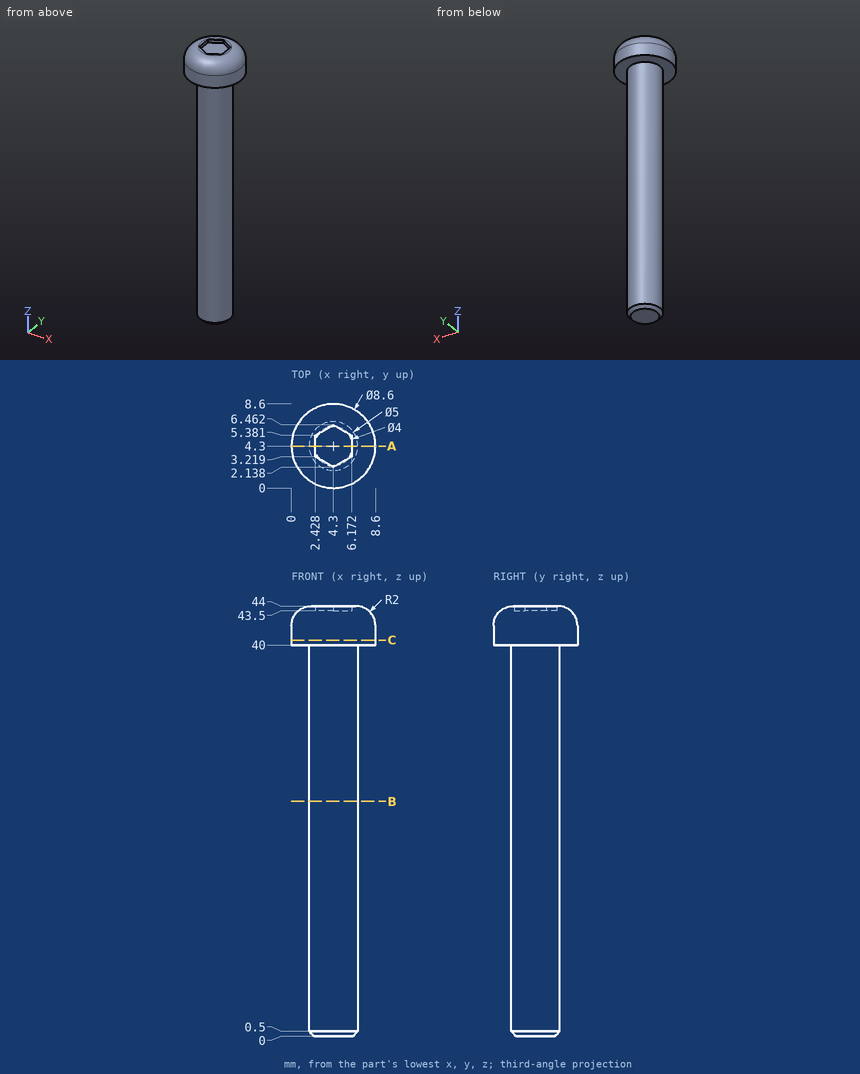
Source: three-view drawing plus pictorial views. Frame: mm from the lowest corner of the part. Coordinates: 2 decimals unless noted, no trailing zeros. Loops run counter-clockwise (first coordinate to the right, second up) from the corner with the lowest first, then second, coordinate; pieces in that order, holes last. Notation, with made-up numbers: (29.25, 22) - (39.25, 22) arc R8 ccw to (39.25, 36) - close; hole circle Ø10 at (82.25, -18). An arc over 180 degrees is marked (long way). One line per question, with ' | ' between items.
1) Section C-C, the plane z = 40.5. Return loops of the section in (x, y), then the cut area to 3 significant figures.
Report:
outline: circle Ø8.6 at (4.3, 4.3) | area: 58.1 mm²
2) Section B-B, the plane z = 24. Return loops of the section in (x, y), then the cut area to 3 significant figures.
Report:
outline: circle Ø5 at (4.3, 4.3) | area: 19.6 mm²
3) Line query: line 1 along Z through (x, y) = (5, 3); line 2 along X through (y, z) = (4.5, 7.5); line 3 along Z through (x, y) = (1.5, 1.75). Output: solid intervals per line, ascending.
Report:
line 1: z = 0 to 43.5 | line 2: x = 1.81 to 6.79 | line 3: z = 40 to 43.34
4) Section A-A, the plane y = 4.3. Return loops of the section in (x, z).
Report:
outline: (0, 40) - (1.8, 40) - (1.8, 0.5) - (2.3, 0) - (6.3, 0) - (6.8, 0.5) - (6.8, 40) - (8.6, 40) - (8.6, 42) arc R2 ccw to (6.6, 44) - (6.17, 44) - (6.17, 43.5) - (2.43, 43.5) - (2.43, 44) - (2, 44) arc R2 ccw to (0, 42) - close
5) First-contact query: P1, Ø3, axis at y = 3.5, z = 12.5, coming from the +X side; P2, Ø1.5, axis at x = 2, y = 5, coming from the -Z side; P3, Ø3, axis at y = 5, z = 22, coming from the -X side; P4, Ø1.9, axis at x = 3.5, y = 4.5, coming from the +Z side. Flat tips, straight axial feed; report the tip coordinate or a pass-through.
Report:
P1: stops at x = 6.8 | P2: stops at z = 0 | P3: stops at x = 1.8 | P4: stops at z = 43.5
